```python
from build123d import *

# Parameters (mm, degrees)
SKETCH1_W               = 1.5
SKETCH1_H               = 33.5
SKETCH1_W_2             = 33.5
SKETCH1_H_2             = 1.5
BOSS_EXTRUDE1_DEPTH     = 210
CUT_EXTRUDE2_DEPTH      = 62
CUT_EXTRUDE2_DEPTH_BACK = 62
CUT_EXTRUDE3_DEPTH      = 62
SKETCH5_R               = 2.75
CUT_EXTRUDE4_DEPTH      = 5
FILLET1_R               = 1
FILLET2_R               = 2
SKETCH6_W               = 37.5
SKETCH6_H               = 1.436491673
CUT_EXTRUDE5_DEPTH      = 5
SKETCH7_W               = 1.5
SKETCH7_H               = 45.359757049
CUT_EXTRUDE6_DEPTH      = 5
SKETCH8_R               = 2.75
CUT_EXTRUDE7_DEPTH      = 5


with BuildPart() as part:
    # Sketch1 → Boss-Extrude1 (new body)
    with BuildSketch(Plane.XY):
        with Locations((0, 0.75)):
            Rectangle(SKETCH1_W, SKETCH1_H)
        with Locations((17.5, -16.75)):
            Rectangle(SKETCH1_W_2, SKETCH1_H_2)
        with Locations((0, -16.75)):
            Rectangle(SKETCH1_W, SKETCH1_H_2)
    extrude(amount=BOSS_EXTRUDE1_DEPTH)

    # Sketch3 → Cut-Extrude2 (cut, two sides)
    with BuildSketch(Plane(origin=(0.75, 0, 0), x_dir=(0, 0, -1), z_dir=(1, 0, 0))) as cut_extrude2_sk:
        Polygon((-140, 17.5), (-140, 0), (-153, -16), (-210, -16), (-210, 17.5), align=None)
        Polygon((0, 0), (-17.5, -16), (-17.5, -36.829348397), (0, -36.829348397), align=None)
    extrude(amount=CUT_EXTRUDE2_DEPTH, mode=Mode.SUBTRACT)
    extrude(cut_extrude2_sk.sketch, amount=-CUT_EXTRUDE2_DEPTH_BACK, mode=Mode.SUBTRACT)

    # Sketch4 → Cut-Extrude3 (cut)
    with BuildSketch(Plane(origin=(0, -16, 0), x_dir=(1, 0, 0), z_dir=(0, 1, 0))):
        Polygon((16.75, -210), (-0.75, -192.5), (-0.75, -210), align=None)
        Polygon((34.25, -70), (16.75, -70), (0.75, -55), (0.75, -17.5), (34.25, -17.5), align=None)
    extrude(amount=-CUT_EXTRUDE3_DEPTH, mode=Mode.SUBTRACT)

    # Sketch5 → Cut-Extrude4 (cut)
    with BuildSketch(Plane(origin=(0.75, 0, 0), x_dir=(0, 0, -1), z_dir=(1, 0, 0))):
        with Locations(Location((-8, 9.5, 0), (0, 0, 90))):
            Circle(SKETCH5_R)
        with Locations(Location((-28, 9.5, 0), (0, 0, 90))):
            Circle(SKETCH5_R)
        with Locations(Location((-48, 9.5, 0), (0, 0, 90))):
            Circle(SKETCH5_R)
        with Locations(Location((-68, 9.5, 0), (0, 0, 90))):
            Circle(SKETCH5_R)
        with Locations(Location((-88, 9.5, 0), (0, 0, 90))):
            Circle(SKETCH5_R)
        with Locations(Location((-108, 9.5, 0), (0, 0, 90))):
            Circle(SKETCH5_R)
        with Locations(Location((-128, 9.5, 0), (0, 0, 90))):
            Circle(SKETCH5_R)
        with Locations(Location((-18, -5.5, 0), (0, 0, 90))):
            Circle(SKETCH5_R)
        with Locations(Location((-38, -5.5, 0), (0, 0, 90))):
            Circle(SKETCH5_R)
        with Locations(Location((-58, -5.5, 0), (0, 0, 90))):
            Circle(SKETCH5_R)
        with Locations(Location((-78, -5.5, 0), (0, 0, 90))):
            Circle(SKETCH5_R)
        with Locations(Location((-98, -5.5, 0), (0, 0, 90))):
            Circle(SKETCH5_R)
        with Locations(Location((-118, -5.5, 0), (0, 0, 90))):
            Circle(SKETCH5_R)
        with Locations(Location((-138, -5.5, 0), (0, 0, 90))):
            Circle(SKETCH5_R)
    extrude(amount=-CUT_EXTRUDE4_DEPTH, mode=Mode.SUBTRACT)

    # Fillet1
    fillet1_edges = [part.edges().sort_by_distance(p)[0] for p in [
        (0.75, -16, 104),
    ]]
    fillet(fillet1_edges, radius=FILLET1_R)

    # Fillet2
    fillet2_edges = [part.edges().sort_by_distance(p)[0] for p in [
        (-0.75, -17.5, 105),
    ]]
    fillet(fillet2_edges, radius=FILLET2_R)

    # Sketch6 → Cut-Extrude5 (cut)
    with BuildSketch(Plane(origin=(0.75, 0, 0), x_dir=(0, 0, -1), z_dir=(1, 0, 0))):
        with Locations((-36.25, -16.718245837)):
            Rectangle(SKETCH6_W, SKETCH6_H)
    extrude(amount=-CUT_EXTRUDE5_DEPTH, mode=Mode.SUBTRACT)

    # Sketch7 → Cut-Extrude6 (cut)
    with BuildSketch(Plane(origin=(0, -16, 0), x_dir=(1, 0, 0), z_dir=(0, 1, 0))):
        with Locations((0.063508327, -175.679878524)):
            Rectangle(SKETCH7_W, SKETCH7_H)
    extrude(amount=-CUT_EXTRUDE6_DEPTH, mode=Mode.SUBTRACT)

    # Sketch8 → Cut-Extrude7 (cut)
    with BuildSketch(Plane(origin=(0, -16, 0), x_dir=(1, 0, 0), z_dir=(0, 1, 0))):
        with Locations(Location((11.25, -72, 0), (0, 0, 270))):
            Circle(SKETCH8_R)
        with Locations(Location((11.25, -92, 0), (0, 0, 270))):
            Circle(SKETCH8_R)
        with Locations(Location((11.25, -112, 0), (0, 0, 270))):
            Circle(SKETCH8_R)
        with Locations(Location((11.25, -132, 0), (0, 0, 270))):
            Circle(SKETCH8_R)
        with Locations(Location((11.25, -152, 0), (0, 0, 270))):
            Circle(SKETCH8_R)
        with Locations(Location((11.25, -172, 0), (0, 0, 270))):
            Circle(SKETCH8_R)
        with Locations(Location((11.25, -192, 0), (0, 0, 270))):
            Circle(SKETCH8_R)
        with Locations(Location((26.25, -82, 0), (0, 0, 270))):
            Circle(SKETCH8_R)
        with Locations(Location((26.25, -102, 0), (0, 0, 270))):
            Circle(SKETCH8_R)
        with Locations(Location((26.25, -122, 0), (0, 0, 270))):
            Circle(SKETCH8_R)
        with Locations(Location((26.25, -142, 0), (0, 0, 270))):
            Circle(SKETCH8_R)
        with Locations(Location((26.25, -162, 0), (0, 0, 270))):
            Circle(SKETCH8_R)
        with Locations(Location((26.25, -182, 0), (0, 0, 270))):
            Circle(SKETCH8_R)
        with Locations(Location((26.25, -202, 0), (0, 0, 270))):
            Circle(SKETCH8_R)
    extrude(amount=-CUT_EXTRUDE7_DEPTH, mode=Mode.SUBTRACT)


solid = part.part
```
Can you work these out from the model? Positions are in its coordinate system, mm. Give positions to 0.01 mm unless a question says otherwise; leave off trailing zeros. Order: outer loops, then holes, each group sorted by start corner. A loop starts at its lowest first (then second) coordinate and runs counter-clockwise, first axis right, second up. Notation, with made-up numbers: (73.5, 70.5) - (102.5, 70.5) arc R10 ccw to (102.5, 88.5) - close; hole circle Ø4 at (51, 1). An arc over 180 degrees is marked (long way). Use a Markdown table: item, result. Add a question column.
Q1. Please list where these lines run through material, in increasing order: line 1 along X through (y, z) = (-17, 182); line 2 along Y through (x, z) = (26, 150.5); line 3 along X through (y, z) = (-16.35, 92).
Q2. If we section it at C-C on x = 18.5: Write out the boundary of the cut face in (y, z), plus the area to 3 significant figures.
Q3. If we section it at D-D on y = 3.5: Write out the boundary of the cut face in (x, z).
Q4. If we section it at A-A on z = 182: Write out the boundary of the cut face in (x, y).
Q5. If we section it at B-B on z = 38: Write out the boundary of the cut face in (x, y), plus the area to 3 significant figures.
Q6. If we mould it in two halves opening along Y, with no side actions, what happens to faces 1 (the flat face through (-0.04, -7.89, 146.41)), 2 (the flat face through (0.01, -7.89, 8.63)), 3 (the cylindrical face through (12.08, -16.74, 154.62)), 4 (the cylindrical face through (0.01, -5.858, 40.727))? For each: released by +Y, released by -Y, zero draft, split by the parting line, or undercut.
Q7. I'm going to push flat-ended pins straight in: pin 1 (1.6 mm diameter, centred on x = 0, y = -17, fed in from -Z); pin 2 (7 mm diameter, centred on y = -5.5, z = 98, fed in from +X); pin 3 (9 mm diameter, centred on x = 26.25, z = 102, fed in from +Y). Where does each tip first touch, or does it pass through?
Answers follow:
| question | item | result |
|---|---|---|
| 1 | line 1 | x = 0.81 to 23.5, 29 to 34.25 |
| 1 | line 2 | y = -17.5 to -16 |
| 1 | line 3 | x = -0.56 to 8.5, 14 to 34.25 |
| 2 | outline | (-17.5, 70) - (-16, 70) - (-16, 210) - (-17.5, 210) - close |
| 2 | area | 210 mm^2 |
| 3 | outline | (-0.75, 0) - (0.75, 0) - (0.75, 140) - (-0.75, 140) - close |
| 4 | outline | (0.81, -17.45) arc R2 ccw to (1.25, -17.5) - (23.5, -17.5) - (23.5, -16) - (0.81, -16) - close; (29, -17.5) - (34.25, -17.5) - (34.25, -16) - (29, -16) - close |
| 5 | outline | (-0.75, -15.5) arc R2 ccw to (-0.69, -16) - (0.75, -16) - (0.75, -8.25) - (-0.75, -8.25) - close; (-0.75, -2.75) - (0.75, -2.75) - (0.75, 17.5) - (-0.75, 17.5) - close |
| 5 | area | 42.0 mm^2 |
| 6 | face 1 | released by +Y |
| 6 | face 2 | released by -Y |
| 6 | face 3 | zero draft |
| 6 | face 4 | undercut |
| 7 | pin 1 | stops at z = 55 |
| 7 | pin 2 | stops at x = 0.75 |
| 7 | pin 3 | stops at y = -16 |
